Autodesk Inventor part; units mm, degrees
ref_plane "YZ Plane" through (0, 0, 0) normal (1, 0, 0) x (0, 1, 0)
ref_plane "XZ Plane" through (0, 0, 0) normal (0, 1, 0) x (-1, 0, 0)
ref_plane "XY Plane" through (0, 0, 0) normal (0, 0, 1) x (1, 0, 0)
sketch "Sketch1" plane through (0, 0, 0) normal (1, 0, 0) x (0, 1, 0)
  point P0 (0, 0)
sketch "Sketch2" plane through (0, 0, 0) normal (1, 0, 0) x (0, 1, 0)
  line L0 (22.3119, 47.1251) -> (-47.5381, 47.1251)
  line L1 (-47.5381, 47.1251) -> (-47.5381, -44.3149)
  line L2 (-47.5381, -44.3149) -> (22.3119, -44.3149)
  line L3 (22.3119, -44.3149) -> (22.3119, 47.1251)
  point P0 (0, 0)
  dimension "d0" = 91.44
  dimension "d1" = 69.85
extrude "Extrusion1" add sketch "Sketch2" along normal blind 6.35
sketch "Sketch3" plane through (6.35, 0, 0) normal (1, 0, 0) x (0, 0, -1)
  line L0 (-47.1251, 22.3119) -> (-47.1251, -47.5381)
  line L1 (-47.1251, -47.5381) -> (-47.1251, 22.3119)
  line L2 (44.3149, -47.5381) -> (44.3149, 22.3119)
  line L3 (-47.1251, 22.3119) -> (44.3149, 22.3119)
  line L4 (44.3149, 22.3119) -> (44.3149, -47.5381)
  line L5 (-47.1251, -47.5381) -> (-40.7751, -47.5381)
  line L6 (-47.1251, -47.5381) -> (44.3149, -47.5381)
  line L7 (37.9649, -47.5381) -> (44.3149, -47.5381)
  line L8 (-40.7751, -47.5381) -> (-34.4251, -47.5381)
  line L9 (37.9649, -47.5381) -> (31.6149, -47.5381)
  line L10 (31.6149, -47.5381) -> (31.6149, -44.3631)
  line L11 (31.6149, -44.3631) -> (37.9649, -44.3631)
  line L12 (-34.4251, -47.5381) -> (-34.4251, -44.3631)
  line L13 (-34.4251, -44.3631) -> (-40.7751, -44.3631)
  line L14 (-40.7751, 15.9619) -> (37.9649, 15.9619)
  line L15 (-40.7751, -33.5681) -> (-40.7751, 15.9619)
  line L16 (37.9649, 15.9619) -> (37.9649, -33.5681)
  line L17 (-40.7751, -44.3631) -> (-40.7751, -39.2831)
  line L18 (-40.7751, -39.2831) -> (-34.4251, -39.2831)
  line L19 (-34.4251, -39.2831) -> (-34.4251, -36.1081)
  line L20 (-34.4251, -36.1081) -> (-40.7751, -36.1081)
  line L21 (-40.7751, -36.1081) -> (-40.7751, -33.5681)
  line L22 (37.9649, -44.3631) -> (37.9649, -39.2831)
  line L23 (37.9649, -39.2831) -> (31.6149, -39.2831)
  line L24 (31.6149, -39.2831) -> (31.6149, -36.1081)
  line L25 (31.6149, -36.1081) -> (37.9649, -36.1081)
  line L26 (37.9649, -36.1081) -> (37.9649, -33.5681)
  point P0 (0, 0)
  dimension "d7" = 78.74
  dimension "d10" = 6.35
  dimension "d11" = 3.175
  dimension "d25" = 3.175
  dimension "d26" = 5.08
  dimension "d27" = 5.08
  dimension "d28" = 3.175
  dimension "d29" = 3.175
  dimension "d30" = 6.35
  dimension "d31" = 66.04
extrude "Extrusion2" add sketch "Sketch3" along normal blind 111.76 contours L3 L2 L6 L10 L11 L22 L23 L24 L25 L26 L16 L14 L15 L21 L20 L19 L18 L17 L13 L12 L5 L0
sketch "Sketch4" plane through (0, 22.3119, 47.1251) normal (0, 1, 0) x (1, 0, 0)
  line L0 (114.935, 6.35) -> (114.935, 85.09)
  line L1 (114.935, 6.35) -> (108.585, 6.35)
  line L2 (108.585, 6.35) -> (108.585, 85.09)
  line L3 (114.935, 85.09) -> (108.585, 85.09)
  point P0 (0, 47.1251)
extrude "Extrusion3" cut sketch "Sketch4" against normal blind 63.5
properties part number "bens capstone"
Could you check a few things on this model? Use its own coordinates, in mm. A direction names the side the tool comes from. Round coordinates to 2 decimals unless told otherwise and drop trailing zeros. Write each loop counter-clockwise with the first axis right and the second up, starting at its lowest first coordinate (ties: lowest second). Pieces come first, ordered by that corner, then holes. Notation, with made-up numbers: (9.5, 1) - (66.5, 1) arc R33 ccw to (66.5, 37) - close; hole circle Ø4 at (89, -2.75). An arc over 180 degrees is marked (long way). Use a Markdown table: item, result.
Q1. I want a section at C-C (z = -35.5). List the corners of the cut face in (x, y) for me (3 decimals), plus the area to 3 significant figures.
Output values:
| item | result |
|---|---|
| outline | (0, -47.538) - (118.11, -47.538) - (118.11, -44.363) - (6.35, -44.363) - (6.35, -39.283) - (108.585, -39.283) - (108.585, -36.108) - (6.35, -36.108) - (6.35, 15.962) - (108.585, 15.962) - (108.585, 22.312) - (0, 22.312) - close; (114.935, -39.283) - (118.11, -39.283) - (118.11, -36.108) - (114.935, -36.108) - close; (114.935, 15.962) - (118.11, 15.962) - (118.11, 22.312) - (114.935, 22.312) - close |
| area | 1,800 mm2 |
Q2. For faces 1 (the flat face through (58, 22.312, 1)), 2 (the flat face through (61, -46, 34.425)), 3 (the flat face through (117, -39.283, 38)), 4 (the flat face through (114.935, -38, -35)), which set-ups out of +Z, -Z, +X, -X, +Y, -Y let a thin tool reach every point of the face, with its end or its side?
Output values:
| item | result |
|---|---|
| face 1 | +Z, -Z, +X, -X, +Y |
| face 2 | +X, -Y |
| face 3 | +X |
| face 4 | +Y |
Q3. Thinking about a two-plate mould opening in X: for faces 5 (the flat face through (108.585, -38, -35)), 6 (the flat face through (58, -12, 47.125)), 7 (the flat face through (118.11, 19, -2)), which applies, released by +X, released by -X, zero draft, split by the parting line, or undercut?
Output values:
| item | result |
|---|---|
| face 5 | undercut |
| face 6 | zero draft |
| face 7 | released by +X |
Q4. For pin 1 (6 mm diameter, centred on x = 31, z = 16, fed in from -Y); pin 2 (2 mm diameter, centred on y = -0.5, z = -7, fed in from +X), each with a flat end and sliding along its axis, tell me the tip position at first contact or that it passes through.
Output values:
| item | result |
|---|---|
| pin 1 | y = 15.96 |
| pin 2 | x = 6.35 |
Q5. Please list where these lines run through material, in increasing order: L1, parallel to Y at x = 24.5, z = -35; L2, parallel to Z at x = 100.5, y = 13.5; L3, parallel to Y at x = 19, z = -12.5.
Output values:
| item | result |
|---|---|
| L1 | -47.54 to -44.36, -39.28 to -36.11, 15.96 to 22.31 |
| L2 | -44.31 to -37.96, 40.78 to 47.13 |
| L3 | 15.96 to 22.31 |
Q6. I want a section at B-B (y = 13). List the corners of the cut face in (x, z) for me, plus the area to 3 significant figures.
Output values:
| item | result |
|---|---|
| outline | (0, -44.31) - (118.11, -44.31) - (118.11, -37.96) - (6.35, -37.96) - (6.35, 40.78) - (118.11, 40.78) - (118.11, 47.13) - (0, 47.13) - close |
| area | 2,000 mm2 |
Q7. I want a section at A-A (z = 12). List the corners of the cut face in (x, y) for me (3 decimals), plus the area to 3 significant figures.
Output values:
| item | result |
|---|---|
| outline | (0, -47.538) - (6.35, -47.538) - (6.35, 15.962) - (108.585, 15.962) - (108.585, 22.312) - (0, 22.312) - close; (114.935, 15.962) - (118.11, 15.962) - (118.11, 22.312) - (114.935, 22.312) - close |
| area | 1,110 mm2 |
Q8. I want a section at D-D (x = 25.5). List the corners of the cut face in (y, z) for me.
Output values:
| item | result |
|---|---|
| outline | (-47.54, -44.31) - (22.31, -44.31) - (22.31, 47.13) - (-47.54, 47.13) - (-47.54, 34.43) - (-44.36, 34.43) - (-44.36, 40.78) - (-39.28, 40.78) - (-39.28, 34.43) - (-36.11, 34.43) - (-36.11, 40.78) - (15.96, 40.78) - (15.96, -37.96) - (-36.11, -37.96) - (-36.11, -31.61) - (-39.28, -31.61) - (-39.28, -37.96) - (-44.36, -37.96) - (-44.36, -31.61) - (-47.54, -31.61) - close |
